Could you check a few things on this model? Use its own coordinates, in mm. Face numbers are marked on the shaded views. Coordinates: 2 decimals unless noted, no trailing zeros. Write each loop counter-clockwise with the first axis right and the second up, starting at its lowest first coordinate (ties: lowest second). Pieces come first, ordered by that corner, then holes. Notation, with made-up numbers: (-39.75, -40) - (12.25, -40) arc R16 ccw to (12.25, -36) - close; hole circle Ø7 at (64, 10). An arc over 180 degrees is marked (long way). Answer as a JSON object with one key per item and string values. Group by question number.
1) If we section it at B-B (y = -68.5): Write out the boundary of the cut face in (x, z) (1 decimal).
2) Please list where these lines run through material, in increasing order: line 1 along Y through (x, z) = (-69.85, -25) (1 decimal); line 2 along Z through (x, y) = (-80.5, -55.5); line 3 along Y through (x, z) = (-72, -43).
3) If we section it at A-A (x = -69.85): Write out the boundary of the cut face in (y, z) (1 decimal), plus the area to 3 significant figures.
4) If we section it at D-D (y = -56.5): Write out the boundary of the cut face in (x, z) (3 decimals).
5) We'd pull the mould along X, two halves only. Please class the marked faces 1, 2 and 3: released by +X, released by -X, zero draft, split by the parting line, or undercut.
6) Will these pins go through, and if not, where does the flat tip stop? pin 1 Ø13.5 at (x, y) = (-69.85, -69.85) entering from +Z; pin 2 Ø5 at (y, z) = (-73.5, -6) entering from +X; pin 3 Ø1.5 at (x, z) = (-65.5, -35.5) entering from +Y; pin 4 Ø1 at (y, z) = (-72, -21) entering from +X.
Autodesk Inventor part; units mm, degrees
ref_plane "YZ Plane" through (0, 0, 0) normal (1, 0, 0) x (0, 1, 0)
ref_plane "XZ Plane" through (0, 0, 0) normal (0, 1, 0) x (-1, 0, 0)
ref_plane "XY Plane" through (0, 0, 0) normal (0, 0, 1) x (1, 0, 0)
sketch "Sketch1" plane through (0, 0, 0) normal (0, 0, 1) x (1, 0, 0)
  circle A0 centre (-69.85, -69.85) radius 15.875
  circle A1 centre (-69.85, -69.85) radius 18.1229
  dimension "d0" = 36.2458
extrude "Extrusion1" add sketch "Sketch1" along normal blind 5.08 contours A0 | A1
sketch "Sketch2" plane through (-69.85, -69.85, 0) normal (0, 0, -1) x (-1, 0, 0)
  circle A0 centre (0, 0) radius 18.1229
  circle A1 centre (0, 0) radius 15.875
  dimension "d3" = 31.75
extrude "Extrusion2" add sketch "Sketch2" along normal blind 55.245 contours A1
sketch "Sketch3" plane through (-69.85, -69.85, 5.08) normal (0, 0, 1) x (1, 0, 0)
  circle A0 centre (0, 0) radius 18.1229
  circle A1 centre (0, 0) radius 11.1125
  dimension "d6" = 22.225
extrude "Extrusion3" cut sketch "Sketch3" against normal through all contours A1
properties part number "Bush bottomplate2"
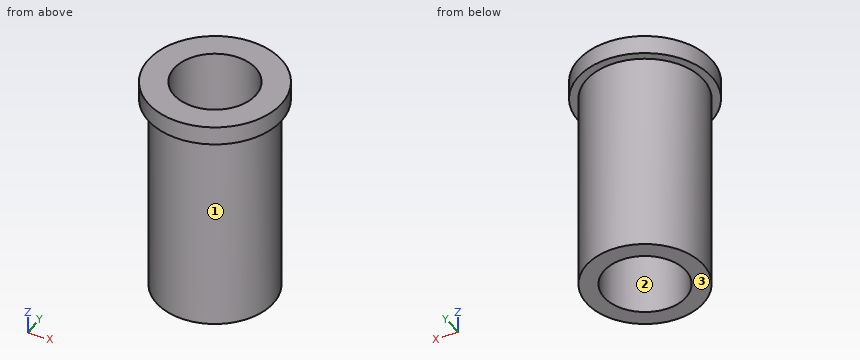
Here are the results:
{
 "1": {"outline": "(-87.9, 0) - (-85.7, 0) - (-85.7, -55.2) - (-80.9, -55.2) - (-80.9, 5.1) - (-87.9, 5.1) - close; (-58.8, -55.2) - (-54, -55.2) - (-54, 0) - (-51.8, 0) - (-51.8, 5.1) - (-58.8, 5.1) - close"},
 "2": {"line 1": "y = -85.7 to -81, -58.7 to -54", "line 2": "z = 0 to 5.08", "line 3": "y = -85.58 to -80.75, -58.95 to -54.12"},
 "3": {"outline": "(-88, 0) - (-85.7, 0) - (-85.7, -55.2) - (-81, -55.2) - (-81, 5.1) - (-88, 5.1) - close; (-58.7, -55.2) - (-54, -55.2) - (-54, 0) - (-51.7, 0) - (-51.7, 5.1) - (-58.7, 5.1) - close", "area": "597 mm²"},
 "4": {"outline": "(-82.106, 0) - (-78.44, 0) - (-78.44, -55.245) - (-61.26, -55.245) - (-61.26, 0) - (-57.594, 0) - (-57.594, 5.08) - (-82.106, 5.08) - close"},
 "5": {"face 1": "split by the parting line", "face 2": "undercut", "face 3": "zero draft"},
 "6": {"pin 1": "passes through", "pin 2": "stops at x = -54.02", "pin 3": "stops at y = -54.39", "pin 4": "stops at x = -54.06"}
}
